```python
from build123d import *

# Parameters (mm, degrees)
F0_R     = 12.7
F1_DEPTH = 25.4
F2_DEPTH = 50.8
F3_R     = 12.7
F4_DEPTH = 25.4


with BuildPart() as f1:
    # F0 (on Front) → F1 (new body)
    with BuildSketch(Plane.XZ):
        with BuildLine():
            ThreePointArc((-25.4, 101.6), (0, 76.2), (25.4, 101.6))
            ThreePointArc((25.4, 101.6), (0, 127), (-25.4, 101.6))
        make_face()
        with Locations((0, 101.6)):
            Circle(F0_R, mode=Mode.SUBTRACT)
        with BuildLine():
            ThreePointArc((-25.4, 0), (0, 25.4), (25.4, 0))
            Line((25.4, 0), (25.4, 101.6))
            ThreePointArc((25.4, 101.6), (0, 76.2), (-25.4, 101.6))
            Line((-25.4, 101.6), (-25.4, 0))
        make_face()
        with BuildLine():
            ThreePointArc((-25.4, 0), (0, -25.4), (25.4, 0))
            ThreePointArc((25.4, 0), (0, 25.4), (-25.4, 0))
        make_face()
        Circle(F0_R, mode=Mode.SUBTRACT)
    extrude(amount=-F1_DEPTH)

    # F0 (on Front) → F2 (join)
    with BuildSketch(Plane.XZ):
        with BuildLine():
            ThreePointArc((-25.4, 0), (0, -25.4), (25.4, 0))
            ThreePointArc((25.4, 0), (0, 25.4), (-25.4, 0))
        make_face()
        Circle(F0_R, mode=Mode.SUBTRACT)
    extrude(amount=F2_DEPTH)

    # F3 (on face) → F4 (join)
    with BuildSketch(Plane.XZ.offset(50.8)):
        with BuildLine():
            ThreePointArc((25.4, 101.6), (0, 127), (-25.4, 101.6))
            ThreePointArc((-25.4, 101.6), (0, 76.2), (25.4, 101.6))
        make_face()
        with Locations((0, 101.6)):
            Circle(F3_R, mode=Mode.SUBTRACT)
        with BuildLine():
            ThreePointArc((25.4, 101.6), (0, 76.2), (-25.4, 101.6))
            Line((-25.4, 101.6), (-25.4, 0))
            ThreePointArc((-25.4, 0), (0, 25.4), (25.4, 0))
            Line((25.4, 0), (25.4, 101.6))
        make_face()
        with BuildLine():
            ThreePointArc((25.4, 0), (0, 25.4), (-25.4, 0))
            ThreePointArc((-25.4, 0), (0, -25.4), (25.4, 0))
        make_face()
        Circle(F3_R, mode=Mode.SUBTRACT)
    extrude(amount=F4_DEPTH)


solid = f1.part
```
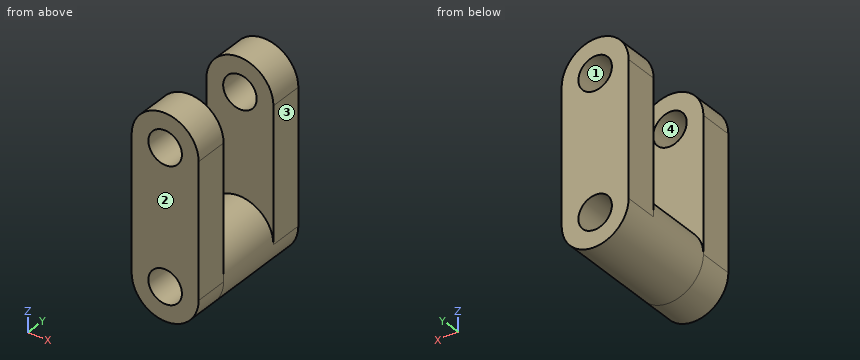
Verification items for the finished model (mm, model axes). Face numbers are marked on the shaded views. Round coordinates to 2 decimals unless told otherwise and drop trailing zeros. Loops run counter-clockwise (first coordinate to the right, second up) from the corner with the lowest first, then second, coordinate; pieces in that order, holes last. Notation, with made-up numbers: (2, 87) -> (13, 87) arc R24 ccw to (13, 106) -> close; hole circle Ø11 at (25.25, 44). An arc over 180 degrees is marked (long way). Answer as a JSON object with one key per item and string values.
Q1. Section check D-D (z = 112). Record the boundary of the cut face in (x, y), then the cut area to 3 significant figures.
Data:
{"outline": "(-23.17, -76.2) -> (-7.29, -76.2) -> (-7.29, -50.8) -> (-23.17, -50.8) -> close; (-23.17, 0) -> (-7.29, 0) -> (-7.29, 25.4) -> (-23.17, 25.4) -> close; (7.29, -76.2) -> (23.17, -76.2) -> (23.17, -50.8) -> (7.29, -50.8) -> close; (7.29, 0) -> (23.17, 0) -> (23.17, 25.4) -> (7.29, 25.4) -> close", "area": "1,610 mm2"}
Q2. Scan lines: line 1 (Z direction, x = 0, y = -68.75); line 2 (Y direction, x = 9.5, z = 60); line 3 (X direction, y = 1, z = 101). Record each from-to range of solid material in increasing order. Write a range as from..to.
Data:
{"line 1": "z = -25.4..-12.7, 12.7..88.9, 114.3..127", "line 2": "y = -76.2..-50.8, 0..25.4", "line 3": "x = -25.4..-12.69, 12.69..25.4"}
Q3. Draft check along X on the marked faces 1, 2, 3 and 4. Enter one of: pulls with the +X half, pulls with the -X half, needs draft (parallel to the pull), parting line crosses it, or undercut.
Data:
{"face 1": "undercut", "face 2": "needs draft", "face 3": "pulls with the +X half", "face 4": "undercut"}
Q4. Section check A-A (x = 0). Record the boundary of the cut face in (y, z), then the cut area to 3 significant figures.
Data:
{"outline": "(-76.2, -25.4) -> (25.4, -25.4) -> (25.4, -12.7) -> (-76.2, -12.7) -> close; (-76.2, 12.7) -> (25.4, 12.7) -> (25.4, 88.9) -> (0, 88.9) -> (0, 25.4) -> (-50.8, 25.4) -> (-50.8, 88.9) -> (-76.2, 88.9) -> close; (-76.2, 114.3) -> (-50.8, 114.3) -> (-50.8, 127) -> (-76.2, 127) -> close; (0, 114.3) -> (25.4, 114.3) -> (25.4, 127) -> (0, 127) -> close", "area": "6,450 mm2"}
Q5. Go/stop test with flat-tipped pins: P1, Ø4, axis at x = 16, y = -48, coming from the -Z side; P2, Ø2, axis at x = -5.5, y = -32, coming from the -Z side; P3, Ø10, axis at y = -42, z = -8, coming from the -X side. Record where each tip stops, or that it passes through.
Data:
{"P1": "stops at z = -21.19", "P2": "stops at z = -25", "P3": "stops at x = -25.22"}
Q6. Section check B-B (y = 9.5). Record the boundary of the cut face in (x, z), then the cut area to 3 significant figures.
Data:
{"outline": "(-25.4, 0) arc R25.4 ccw to (25.4, 0) -> (25.4, 101.6) arc R25.4 ccw to (-25.4, 101.6) -> close; hole circle Ø25.4 at (0, 0); hole circle Ø25.4 at (0, 101.6)", "area": "6,170 mm2"}
Q7. Section check C-C (z = 79). Record the boundary of the cut face in (x, y).
Data:
{"outline": "(-25.4, -76.2) -> (25.4, -76.2) -> (25.4, -50.8) -> (-25.4, -50.8) -> close; (-25.4, 0) -> (25.4, 0) -> (25.4, 25.4) -> (-25.4, 25.4) -> close"}
